```python
from build123d import *

# Parameters (mm, degrees)
BOSS_EXTRUDE1_DEPTH      = 10
BOSS_EXTRUDE2_DEPTH      = 10
BOSS_EXTRUDE2_DEPTH_BACK = 160
SKETCH4_R                = 2.5
CUT_EXTRUDE2_DEPTH       = 2.5
FILLET1_R                = 2
BOSS_EXTRUDE6_DEPTH      = 2.5
BOSS_EXTRUDE7_DEPTH      = 3
SKETCH8_W                = 2.5
SKETCH8_H                = 3
BOSS_EXTRUDE8_DEPTH      = 47
SKETCH9_R                = 2.5
CUT_EXTRUDE3_DEPTH       = 344.969838794
SKETCH10_W               = 3
SKETCH10_H               = 150
BOSS_EXTRUDE9_DEPTH      = 0.5
FILLET2_R                = 2
SKETCH11_W               = 7.5
SKETCH11_H               = 3
BOSS_EXTRUDE10_DEPTH     = 10
SKETCH12_R               = 1.5
CUT_EXTRUDE4_DEPTH       = 10


with BuildPart() as part:
    # Sketch3 → Boss-Extrude1 (new body)
    with BuildSketch(Plane(origin=(0, 0, 0), x_dir=(1, 0, 0), z_dir=(0, 1, 0))):
        Polygon((50, 85), (50, 150), (0, 150), (0, 0), (50, 0), (50, 65), (140, 65), (140, 0), (160, 0), (160, 65), (250, 65), (250, 0), (300, 0), (300, 150), (250, 150), (250, 85), (160, 85), (160, 150), (140, 150), (140, 85), align=None)
    extrude(amount=-BOSS_EXTRUDE1_DEPTH)

    # Sketch4 → Boss-Extrude2 (add, two sides: drawn at the far end of the back side and taken through both)
    with BuildSketch(Plane.XY.offset(-BOSS_EXTRUDE2_DEPTH_BACK)):
        with Locations((250, 0)):
            Circle(SKETCH4_R)
    extrude(amount=BOSS_EXTRUDE2_DEPTH + BOSS_EXTRUDE2_DEPTH_BACK)

    # Sketch5 → Cut-Extrude2 (cut)
    with BuildSketch(Plane(origin=(0, 0, 0), x_dir=(1, 0, 0), z_dir=(0, 1, 0))):
        Polygon((44, 144), (6, 144), (6, 6), (44, 6), (44, 71), (146, 71), (146, 6), (154, 6), (154, 71), (241.5, 71), (241.5, 79), (154, 79), (154, 144), (146, 144), (146, 79), (44, 79), align=None)
    extrude(amount=-CUT_EXTRUDE2_DEPTH, mode=Mode.SUBTRACT)

    # Fillet1
    fillet1_edges = [part.edges().sort_by_distance(p)[0] for p in [
        (95, -2.5, -71),
        (44, -2.5, -38.5),
        (25, -2.5, -6),
        (6, -2.5, -75),
        (25, -2.5, -144),
        (44, -2.5, -111.5),
        (95, -2.5, -79),
        (146, -2.5, -111.5),
        (150, -2.5, -144),
        (154, -2.5, -111.5),
        (197.75, -2.5, -79),
        (241.5, -2.5, -75),
        (197.75, -2.5, -71),
        (154, -2.5, -38.5),
        (150, -2.5, -6),
        (146, -2.5, -38.5),
    ]]
    fillet(fillet1_edges, radius=FILLET1_R)

    # Sketch6 → Boss-Extrude6 (add)
    with BuildSketch(Plane.XY):
        with BuildLine():
            Line((297, 3), (297, 0))
            Line((297, 0), (297.5, 0))
            ThreePointArc((297.5, 0), (300, 2.5), (302.5, 0))
            ThreePointArc((302.5, 0), (301.767766953, -1.767766953), (300, -2.5))
            Line((300, -2.5), (300, -3))
            Line((300, -3), (303, -3))
            Line((303, -3), (303, 3))
            Line((303, 3), (297, 3))
        make_face()
        with BuildLine():
            Line((297.5, 0), (297, 0))
            Line((297, 0), (252.5, 0))
            ThreePointArc((252.5, 0), (251.767766953, -1.767766953), (250, -2.5))
            Line((250, -2.5), (250, -10))
            Line((250, -10), (300, -10))
            Line((300, -10), (300, -3))
            Line((300, -3), (300, -2.5))
            ThreePointArc((300, -2.5), (298.232233047, -1.767766953), (297.5, 0))
        make_face()
    boss_extrude6 = extrude(amount=BOSS_EXTRUDE6_DEPTH)

    # Mirror2: Boss-Extrude6 across plane
    add(boss_extrude6.mirror(Plane.XY.offset(-75)))

    # Sketch7 → Boss-Extrude7 (add)
    with BuildSketch(Plane(origin=(300, 0, 0), x_dir=(0, 0, -1), z_dir=(1, 0, 0))):
        Polygon((0, -3), (150, -3), (152.5, -3), (152.5, -10), (-2.5, -10), (-2.5, -3), align=None)
    extrude(amount=BOSS_EXTRUDE7_DEPTH)

    # Sketch8 → Boss-Extrude8 (add)
    with BuildSketch(Plane.ZY.offset(-297)):
        with Locations((1.25, 1.5)):
            Rectangle(SKETCH8_W, SKETCH8_H)
    boss_extrude8 = extrude(amount=BOSS_EXTRUDE8_DEPTH)

    # Mirror3: Boss-Extrude8 across plane
    add(boss_extrude8.mirror(Plane.XY.offset(-75)))

    # Sketch9 → Cut-Extrude3 (cut, through all)
    with BuildSketch(Plane.XY.offset(2.5)):
        with Locations((300, 0)):
            Circle(SKETCH9_R)
    extrude(amount=-CUT_EXTRUDE3_DEPTH, mode=Mode.SUBTRACT)

    # Sketch10 → Boss-Extrude9 (add)
    with BuildSketch(Plane(origin=(0, -3, 0), x_dir=(1, 0, 0), z_dir=(0, 1, 0))):
        with Locations((301.5, 75)):
            Rectangle(SKETCH10_W, SKETCH10_H)
    extrude(amount=BOSS_EXTRUDE9_DEPTH)

    # Fillet2
    fillet2_edges = [part.edges().sort_by_distance(p)[0] for p in [
        (50, -10, -32.5),
        (95, -10, -65),
        (275, -10, 2.5),
        (140, -10, -32.5),
        (275, -10, -152.5),
        (150, -10, 0),
        (303, -10, -75),
        (160, -10, -32.5),
        (205, -10, -65),
        (250, -10, -32.5),
        (250, -10, -117.5),
        (25, -10, 0),
        (205, -10, -85),
        (160, -10, -117.5),
        (150, -10, -150),
        (140, -10, -117.5),
        (95, -10, -85),
        (50, -10, -117.5),
        (25, -10, -150),
        (0, -10, -75),
    ]]
    fillet(fillet2_edges, radius=FILLET2_R)

    # Sketch11 → Boss-Extrude10 (add)
    with BuildSketch(Plane(origin=(0, -2.5, 0), x_dir=(1, 0, 0), z_dir=(0, 1, 0))):
        with Locations((25, 75)):
            Rectangle(SKETCH11_W, SKETCH11_H)
    extrude(amount=BOSS_EXTRUDE10_DEPTH)

    # Sketch12 → Cut-Extrude4 (cut)
    with BuildSketch(Plane.XY.offset(-73.5)):
        with Locations((25, 4.5)):
            Circle(SKETCH12_R)
        with BuildLine():
            Line((28.75, -2.5), (27.723784263, 4.878812998))
            ThreePointArc((27.723784263, 4.878812998), (25, 7.25), (22.276215737, 4.878812998))
            Line((22.276215737, 4.878812998), (21.25, -2.5))
            Line((21.25, -2.5), (21.25, 7.5))
            Line((21.25, 7.5), (28.75, 7.5))
            Line((28.75, 7.5), (28.75, -2.5))
        make_face()
    extrude(amount=-CUT_EXTRUDE4_DEPTH, mode=Mode.SUBTRACT)


solid = part.part
```
Verification items for the finished model (mm, model axes). A direction names the side the tool comes from. Round coordinates to 2 decimals unless told otherwise and drop trailing zeros. Order: outer loops, then holes, each group sorted by start corner. A loop starts at its lowest first (then second) coordinate and runs counter-clockwise, first axis right, second up. Notation, with made-up numbers: (41.25, 89) - (97.25, 89) arc R27 ccw to (97.25, 113) - close; hole circle Ø6 at (37, -16.5). An arc over 180 degrees is marked (long way). Use CSV: the item, a comma, the result in double quotes.
(1) Section check B-B on x = 167. Record the boundary of the cut face in (y, z), and give its area (3 significant figures).
Entries:
outline,"(-10, -83) arc R2 ccw to (-8, -85) - (0, -85) - (0, -79) - (-0.5, -79) arc R2 cw to (-2.5, -77) - (-2.5, -73) arc R2 cw to (-0.5, -71) - (0, -71) - (0, -65) - (-8, -65) arc R2 ccw to (-10, -67) - close"
area,"180 mm^2"
(2) Thickness scan on probe 1 along X at (y, z) = (-4.5, -10.5); probe 2 along Z at (x, y) = (178.5, -1); probe 3 along Y at (x, z) = (300, -42.5). Record the ranges inside material, lowest first. Write a range as from..to.
Entries:
probe 1,"0..50, 140..160, 250..303"
probe 2,"-85..-78.94, -71.06..-65"
probe 3,"-10..-2.5"
(3) Gauge pin test, flat ends, axial feed: pin 1 Ø1.7 at (x, y) = (270.5, 0.5) entering from -Z; pin 2 Ø8 at (x, y) = (117, -4.5) entering from +Z; pin 3 Ø2 at (y, z) = (2, -38.5) entering from +X. Record the tip position at first contact, or that the pin passes through.
Entries:
pin 1,"z = -152.5"
pin 2,"z = -65"
pin 3,"x = 252.29"
(4) Section check A-A on z = -135. State how many separate pieces and enclosed holes the cut face has, and give its area (3 significant figures).
Entries:
separate pieces,"3"
enclosed holes,"0"
area,"1,120 mm^2"
(5) Access from +Z, -Z, +X, -X, +Y, -Y to the whole of each face (thin tool, end or side, straight path). Record for faces 1 (the face through (25, -4, 0)), 2 (the face through (25, 1, -73.5)), 3 (the face through (277, 1, 0)).
Entries:
face 1,"+Z, -X, +Y, -Y"
face 2,"+Y"
face 3,"+X, +Y"
